Source: three-view drawing plus pictorial views. Frame: mm from the lowest corner of the part. Round coordinates to 2 decimals unless told otherwise and drop trailing zeros. Loops run counter-clockwise (first coordinate to the right, second up) from the corner with the lowest first, then second, coordinate; pieces in that order, holes last. Notation, with made-up numbers: (83.25, 75.5) -> (119.25, 75.5) arc R9 cw to (119.25, 88.5) -> close; hole circle Ø11 at (79.5, -14). An arc over 180 degrees is marked (long way). Put each result on its own line as item: value. Start each with the question number.
1. Draft query along Z for the marked faces 1, 2 and 3. Return one class per face: pulls with the +Z half, pulls with the -Z half, needs draft (parallel to the pull), parting line crosses it, or undercut.
2. Material intervals for L1, parallel to Y at x = 31, z = 39.5 (3 decimals); L2, parallel to Y at x = 7, z = 57.5, sorted ascending.
3. Cut plane A-A (y = 40). Return the cut outline in (x, z).
4. Cut plane C-C (x = 29.5). Return the cut outline in (y, z), then the cut area to 3 significant figures.
5. Cut plane B-B (z = 40). Return the cut outline in (x, y), then the cut area to 3 significant figures.
6. Contact query for flat-ended pins moving along their axis: pin 1 (12 mm diameter, centred on x = 43, y = 67, fed in from +Z); pin 2 (5 mm diameter, centred on x = 29.5, y = 52.5, fed in from -Z); pin 3 (8 mm diameter, centred on x = 45, y = 23, fed in from +Z). Output: stop coordinate, or through.
7. Cut plane D-D (x = 51). Return the cut outline in (y, z), then the cut area to 3 significant figures.
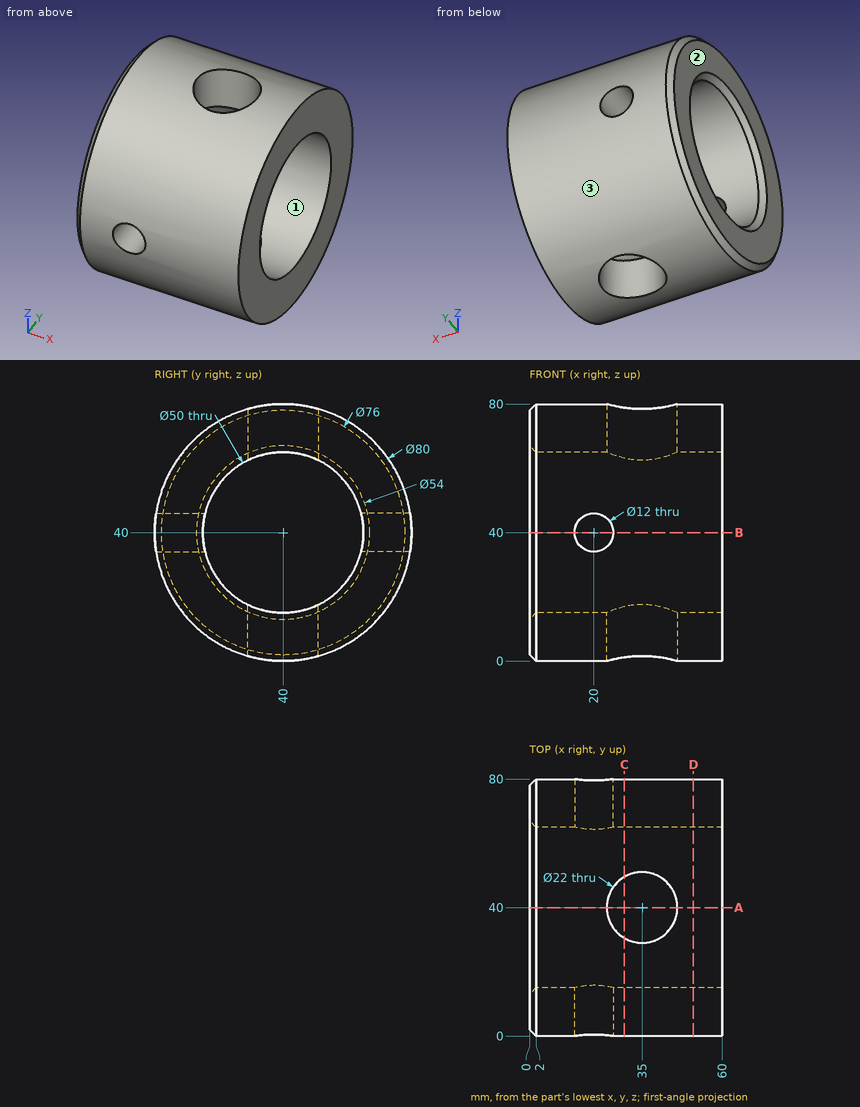
Solution:
1. face 1: undercut
1. face 2: needs draft
1. face 3: parting line crosses it
2. L1: y = 0.003 to 15.005, 64.995 to 79.997
2. L2: y = 4.03 to 22.15, 57.85 to 75.97
3. outline: (0, 2) -> (2, 0) -> (24, 0) -> (24, 15) -> (2, 15) -> (0, 13) -> close; (0, 67) -> (2, 65) -> (24, 65) -> (24, 80) -> (2, 80) -> (0, 78) -> close; (46, 0) -> (60, 0) -> (60, 15) -> (46, 15) -> close; (46, 65) -> (60, 65) -> (60, 80) -> (46, 80) -> close
4. outline: (30.47, 1.15) -> (30.47, 16.89) arc R25 cw to (30.47, 63.11) -> (30.47, 78.85) arc R40 ccw to start; (49.53, 1.15) arc R40 ccw to (49.53, 78.85) -> (49.53, 63.11) arc R25 cw to (49.53, 16.89) -> close
4. area: 2,480 mm^2
5. outline: (0, 2) -> (2, 0) -> (14, 0) -> (14, 15) -> (2, 15) -> (0, 13) -> close; (0, 67) -> (2, 65) -> (14, 65) -> (14, 80) -> (2, 80) -> (0, 78) -> close; (26, 0) -> (60, 0) -> (60, 15) -> (26, 15) -> close; (26, 65) -> (60, 65) -> (60, 80) -> (26, 80) -> close
5. area: 1,430 mm^2
6. pin 1: stops at z = 74.04
6. pin 2: stops at z = 1.27
6. pin 3: stops at z = 77.83
7. outline: circle Ø80 at (40, 40); hole circle Ø50 at (40, 40)
7. area: 3,060 mm^2
